```python
from build123d import *

# Parameters (mm, degrees)
SKETCH1_R                      = 2.55
SKETCH1_R_2                    = 11
BASE_DEPTH                     = 5
SKETCH1_3_R                    = 15
SKETCH1_3_R_2                  = 11
STEM_DEPTH                     = 150
RIBS_DEPTH                     = 2
CIRPATTERN1_COUNT              = 4
SKETCH4_W                      = 90.4
SKETCH4_H                      = 80
TOP_PLATE_DEPTH                = 10
SKETCH6_W                      = 90.4
SKETCH6_H                      = 10
BOSS_EXTRUDE7_DEPTH            = 19
RIB1_START                     = -2.5
RIB1_DEPTH                     = 5
CIRPATTERN6_COUNT              = 4
CUT_EXTRUDE1_REACH             = 170.039
SKETCH10_R                     = 2.4
CUT_EXTRUDE1_DIRECTION_2_DEPTH = 169.039429897
FILLET1_R                      = 10
FILLET2_R                      = 10
SKETCH13_W                     = 5
SKETCH13_H                     = 25.209800542
BOSS_EXTRUDE10_DEPTH           = 140
BOSS_EXTRUDE11_DEPTH           = 141
BOSS_EXTRUDE11_START           = -9.462383487
BOSS_EXTRUDE11_2_DEPTH         = 9.462383487
BOSS_EXTRUDE11_START_2         = -22
BOSS_EXTRUDE11_3_OUTLINE_W     = 26
BOSS_EXTRUDE11_3_OUTLINE_H     = 36
BOSS_EXTRUDE11_3_DEPTH         = 10.305131811
SKETCH16_W                     = 125.849741583
SKETCH16_H                     = 86.760976346
CUT_EXTRUDE2_DEPTH             = 169.039429897


with BuildPart() as part:
    # Sketch1 → base (new body)
    with BuildSketch(Plane(origin=(0, 0, 0), x_dir=(1, 0, 0), z_dir=(0, 1, 0))):
        with BuildLine():
            Line((-16, 25.377155081), (-42.833333333, 8.459051694))
            ThreePointArc((-42.833333333, 8.459051694), (-47.5, 0), (-42.833333333, -8.459051694))
            Line((-42.833333333, -8.459051694), (-16, -25.377155081))
            ThreePointArc((-16, -25.377155081), (0, -30), (16, -25.377155081))
            Line((16, -25.377155081), (42.833333333, -8.459051694))
            ThreePointArc((42.833333333, -8.459051694), (47.5, 0), (42.833333333, 8.459051694))
            Line((42.833333333, 8.459051694), (16, 25.377155081))
            ThreePointArc((16, 25.377155081), (0, 30), (-16, 25.377155081))
        make_face()
        with Locations(Location((-37.5, 0, 0), (0, 0, 270))):
            Circle(SKETCH1_R, mode=Mode.SUBTRACT)
        with Locations(Location((37.5, 0, 0), (0, 0, 270))):
            Circle(SKETCH1_R, mode=Mode.SUBTRACT)
        with Locations(Location((0, 0, 0), (0, 0, 270))):
            Circle(SKETCH1_R_2, mode=Mode.SUBTRACT)
    extrude(amount=BASE_DEPTH)

    # Sketch1<3> → stem (add)
    with BuildSketch(Plane(origin=(0, 0, 0), x_dir=(1, 0, 0), z_dir=(0, 1, 0))):
        with Locations(Location((0, 0, 0), (0, 0, 270))):
            Circle(SKETCH1_3_R)
        with Locations(Location((0, 0, 0), (0, 0, 270))):
            Circle(SKETCH1_3_R_2, mode=Mode.SUBTRACT)
    extrude(amount=STEM_DEPTH)

    # Sketch2 → ribs (add, symmetric)
    with BuildSketch(Plane(origin=(0, 0, 0), x_dir=(0, 0, -1), z_dir=(1, 0, 0))):
        Polygon((-13, 5), (-29, 5), (-13, 45), align=None)
    ribs = extrude(amount=RIBS_DEPTH, both=True)

    # CirPattern1: ribs ×4 about axis
    cirpattern1_axis = Axis((0, 0, 0), (0, 1, 0))
    for i in range(1, CIRPATTERN1_COUNT):
        add(ribs.rotate(cirpattern1_axis, i * 360 / CIRPATTERN1_COUNT))

    # Sketch4 → top plate (add)
    with BuildSketch(Plane(origin=(0, 150, 0), x_dir=(1, 0, 0), z_dir=(0, 1, 0))):
        Rectangle(SKETCH4_W, SKETCH4_H)
    extrude(amount=-TOP_PLATE_DEPTH)

    # Sketch6 → Boss-Extrude7 (add)
    with BuildSketch(Plane.XY.offset(40)):
        with Locations((0, 145)):
            Rectangle(SKETCH6_W, SKETCH6_H)
    extrude(amount=BOSS_EXTRUDE7_DEPTH)

    # Rib1: read off the stored shape, not the designer's step
    # Rib1 outline → Rib1 (add)
    with BuildSketch(Plane(origin=(0, 0, 0), x_dir=(0, 0, -1), z_dir=(1, 0, 0)).offset(RIB1_START)):
        Polygon((-15, 110), (-14.790199458, 110), (-14.790199458, 140), (-40, 140), align=None)
    rib1 = extrude(amount=RIB1_DEPTH)

    # CirPattern6: Rib1 ×4 about axis
    cirpattern6_axis = Axis((0, 0, 0), (0, 1, 0))
    for i in range(1, CIRPATTERN6_COUNT):
        add(rib1.rotate(cirpattern6_axis, i * 360 / CIRPATTERN6_COUNT))

    # Sketch10 → Cut-Extrude1 (cut, up to next)
    with BuildSketch(Plane(origin=(0, 150, 0), x_dir=(1, 0, 0), z_dir=(0, 1, 0)), mode=Mode.PRIVATE) as cut_extrude1_sk1:
        with Locations(Location((35.2, -49, 0), (0, 0, 90))):
            Circle(SKETCH10_R)
    cut_extrude1_tool1 = extrude(cut_extrude1_sk1.sketch, amount=-CUT_EXTRUDE1_REACH, mode=Mode.PRIVATE) & part.part
    # Sketch10 → Cut-Extrude1 (cut, up to next)
    with BuildSketch(Plane(origin=(0, 150, 0), x_dir=(1, 0, 0), z_dir=(0, 1, 0)), mode=Mode.PRIVATE) as cut_extrude1_sk2:
        with Locations(Location((-35.2, -49, 0), (0, 0, 90))):
            Circle(SKETCH10_R)
    cut_extrude1_tool2 = extrude(cut_extrude1_sk2.sketch, amount=-CUT_EXTRUDE1_REACH, mode=Mode.PRIVATE) & part.part
    add(cut_extrude1_tool1.solids().sort_by_distance((35.2, 150, 49))[0], mode=Mode.SUBTRACT)
    add(cut_extrude1_tool2.solids().sort_by_distance((-35.2, 150, 49))[0], mode=Mode.SUBTRACT)

    # Sketch10 → Cut-Extrude1 direction 2 (cut)
    with BuildSketch(Plane(origin=(0, 150, 0), x_dir=(1, 0, 0), z_dir=(0, 1, 0))):
        with Locations(Location((35.2, -49, 0), (0, 0, 90))):
            Circle(SKETCH10_R)
        with Locations(Location((-35.2, -49, 0), (0, 0, 90))):
            Circle(SKETCH10_R)
    extrude(amount=CUT_EXTRUDE1_DIRECTION_2_DEPTH, mode=Mode.SUBTRACT)

    # Fillet1
    fillet1_edges = [part.edges().sort_by_distance(p)[0] for p in [
        (-45.2, 145, 59),
    ]]
    fillet(fillet1_edges, radius=FILLET1_R)

    # Fillet2
    fillet2_edges = [part.edges().sort_by_distance(p)[0] for p in [
        (45.2, 145, 59),
    ]]
    fillet(fillet2_edges, radius=FILLET2_R)

    # Sketch13 → Boss-Extrude10 (add, through all)
    with BuildSketch(Plane.XZ.offset(-140)):
        with Locations((0, -27.395099729)):
            Rectangle(SKETCH13_W, SKETCH13_H)
    extrude(amount=BOSS_EXTRUDE10_DEPTH)

    # Boss-Extrude11: read off the stored shape, not the designer's step
    # Boss-Extrude11 outline → Boss-Extrude11 (add)
    with BuildSketch(Plane(origin=(0, 0, 0), x_dir=(1, 0, 0), z_dir=(0, 1, 0))):
        with BuildLine():
            ThreePointArc((2.5, 14.790199458), (7.779960403, 12.824672164), (11.962383487, 9.049938193))
            Line((11.962383487, 9.049938193), (2.5, 40))
            Line((2.5, 40), (2.5, 14.790199458))
        make_face()
        with BuildLine():
            ThreePointArc((-11.962383487, 9.049938193), (-7.779960403, 12.824672164), (-2.5, 14.790199458))
            Line((-2.5, 14.790199458), (-2.5, 40))
            Line((-2.5, 40), (-11.962383487, 9.049938193))
        make_face()
    extrude(amount=BOSS_EXTRUDE11_DEPTH)

    # Boss-Extrude11 2 outline → Boss-Extrude11 2 (add)
    with BuildSketch(Plane(origin=(0, 0, 0), x_dir=(1, 0, 0), z_dir=(0, 1, 0)).offset(BOSS_EXTRUDE11_START)):
        with BuildLine():
            Line((-2.5, 40), (-11.962383487, 9.049938193))
            ThreePointArc((-11.962383487, 9.049938193), (0, 15), (11.962383487, 9.049938193))
            Line((11.962383487, 9.049938193), (2.5, 40))
            Line((2.5, 40), (-2.5, 40))
        make_face()
    extrude(amount=BOSS_EXTRUDE11_2_DEPTH)

    # Boss-Extrude11 3 outline → Boss-Extrude11 3 (cut)
    with BuildSketch(Plane(origin=(0, 0, 0), x_dir=(1, 0, 0), z_dir=(0, 0.9563047559630354, 0.2923717047227371)).offset(BOSS_EXTRUDE11_START_2)):
        with Locations((0, 22)):
            Rectangle(BOSS_EXTRUDE11_3_OUTLINE_W, BOSS_EXTRUDE11_3_OUTLINE_H)
    extrude(amount=BOSS_EXTRUDE11_3_DEPTH, mode=Mode.SUBTRACT)

    # Sketch16 → Cut-Extrude2 (cut, through all)
    with BuildSketch(Plane.XY):
        with Locations((6.783470695, -43.380488173)):
            Rectangle(SKETCH16_W, SKETCH16_H)
    extrude(amount=-CUT_EXTRUDE2_DEPTH, mode=Mode.SUBTRACT)


solid = part.part
```
Input: part model. Units: mm. Frame: model coordinates. A direction names the side the tool comes from. Give positions to 0.01 mm unless a question says otherwise; leave off trailing zeros. Loops run counter-clockwise (first coordinate to the right, second up) from the corner with the lowest first, then second, coordinate; pieces in that order, holes last. Notation, with made-up numbers: (-22.5, 65) -> (3.5, 65) arc R21 cw to (3.5, 93) -> close; hole circle Ø8 at (-2, 59.25). An arc over 180 degrees is marked (long way). Use a Markdown table: item, result.
Q1. Section query C-C, the plane x = -9. Return the cut outline in (y, z).
Entries:
| item | result |
|---|---|
| outline | (0, -28.62) -> (5, -28.62) -> (5, -18.74) -> (140, -18.74) -> (140, -40) -> (150, -40) -> (150, 59) -> (140, 59) -> (140, 12) -> (5, 12) -> (5, 28.62) -> (0, 28.62) -> (0, 6.32) -> (140, 6.32) -> (140, -6.32) -> (0, -6.32) -> close |
Q2. Access query for faces 1 (the cylindrical face through (40.03, 2.46, -0.33)), 2 (the flat face through (19, 15, -2)), 3 (the flat face through (-27.675, 125.21, -0.035)), 4 (the flat face through (2, 15, 19)), 5 (the cylindrical face through (0, 2, 30)). Directions: +Z, -Z, +X, -X, +Y, -Y. A direction counts if a zero-diameter tool reaches every point of the face in a straight line with its end or side. Return the directions, or none.
Entries:
| item | result |
|---|---|
| face 1 | -Y |
| face 2 | -Z, +X |
| face 3 | +Z, -Z, -X |
| face 4 | +Z, +X |
| face 5 | +Z, -Y |
Q3. Section query B-B, the plane x = 22. Return the cut outline in (y, z), plus the area to 3 significant figures.
Entries:
| item | result |
|---|---|
| outline | (0, -21.59) -> (5, -21.59) -> (5, -2) -> (22.5, -2) -> (22.5, 2) -> (5, 2) -> (5, 21.59) -> (0, 21.59) -> close; (118.4, -2.5) -> (140, -2.5) -> (140, -40) -> (150, -40) -> (150, 59) -> (140, 59) -> (140, 2.5) -> (118.4, 2.5) -> close |
| area | 1,380 mm² |
Q4. Ray query, probe 1 along X at (y, z) = (3, 0); probe 2 along X at (y, z) = (145, 49); probe 3 along Y at (x, z) = (31.5, -6). Return the intervals inside material, ascending. Write a range as from..to.
Entries:
| item | result |
|---|---|
| probe 1 | x = -47.5..-40.05, -34.95..-11, 11..34.95, 40.05..47.5 |
| probe 2 | x = -45.2..-37.6, -32.8..32.8, 37.6..45.2 |
| probe 3 | y = 0..5, 140..150 |
Q5. First-contact query: P1, Ø1.5, axis at x = -14, y = 42.5, coming from the +Z side; P2, Ø8, axis at x = -9.5, y = 98, coming from the +Z side; P3, Ø12, axis at y = 45.5, z = 6, coming from the +X side; P4, Ø4, axis at x = 35.2, z = 49, coming from the -Y side. Flat tips, straight axial feed; report the tip coordinate or a pass-through.
Entries:
| item | result |
|---|---|
| P1 | stops at z = 7.03 |
| P2 | stops at z = 13.96 |
| P3 | stops at x = 15 |
| P4 | passes through |
Q6. Section query D-D, the plane y = 35. Return the cut outline in (x, z).
Entries:
| item | result |
|---|---|
| outline | (-17, -2) -> (-14.87, -2) arc R15 ccw to (-11.96, -9.05) -> (-2.5, -40) -> (2.5, -40) -> (11.96, -9.05) arc R15 ccw to (14.87, -2) -> (17, -2) -> (17, 2) -> (14.87, 2) arc R15 ccw to (2, 14.87) -> (2, 17) -> (-2, 17) -> (-2, 14.87) arc R15 ccw to (-14.87, 2) -> (-17, 2) -> close; hole circle Ø22 at (0, 0) |
Q7. Pull-direction query (Y, two-part tool) for faces 6 (the flat face through (25, 129, 2.5)), 7 (the flat face through (-11, 0, -5)), 8 (the cylindrical face through (-42.35, 145.07, 55.99)); classes: pulls with the +Y half, pulls with the -Y half, needs draft (parallel to the pull), parting line crosses it, or undercut.
Entries:
| item | result |
|---|---|
| face 6 | undercut |
| face 7 | pulls with the -Y half |
| face 8 | needs draft |
Q8. Section query A-A, the plane y = 16.5. Return the cut outline in (x, z).
Entries:
| item | result |
|---|---|
| outline | (-24.4, -2) -> (-14.87, -2) arc R15 ccw to (-11.96, -9.05) -> (-2.5, -40) -> (2.5, -40) -> (11.96, -9.05) arc R15 ccw to (14.87, -2) -> (24.4, -2) -> (24.4, 2) -> (14.87, 2) arc R15 ccw to (2, 14.87) -> (2, 24.4) -> (-2, 24.4) -> (-2, 14.87) arc R15 ccw to (-14.87, 2) -> (-24.4, 2) -> close; hole circle Ø22 at (0, 0) |
